from build123d import *

# Parameters (mm, degrees)
CROQUIS2_W              = 31
CROQUIS2_H              = 130
SALIENTE_EXTRUIR1_DEPTH = 69
CROQUIS3_W              = 130
CROQUIS3_H              = 40
SALIENTE_EXTRUIR2_DEPTH = 715
CROQUIS4_W              = 31
CROQUIS4_H              = 130
SALIENTE_EXTRUIR3_DEPTH = 29
CROQUIS7_W              = 684
CROQUIS7_H              = 20
CORTAR_EXTRUIR2_DEPTH   = 125
CROQUIS8_W              = 684
CROQUIS8_H              = 39.960038326
CORTAR_EXTRUIR3_DEPTH   = 1
REDONDEO1_R             = 4


with BuildPart() as part:
    # Croquis2 → Saliente-Extruir1 (new body)
    with BuildSketch(Plane(origin=(0, 0, 0), x_dir=(1, 0, 0), z_dir=(0, 1, 0))):
        with Locations((15.5, 65)):
            Rectangle(CROQUIS2_W, CROQUIS2_H)
    extrude(amount=SALIENTE_EXTRUIR1_DEPTH)

    # Croquis3 → Saliente-Extruir2 (add)
    with BuildSketch(Plane(origin=(31, 0, 0), x_dir=(0, 0, -1), z_dir=(1, 0, 0))):
        with Locations((65, 20)):
            Rectangle(CROQUIS3_W, CROQUIS3_H)
    extrude(amount=SALIENTE_EXTRUIR2_DEPTH)

    # Croquis4 → Saliente-Extruir3 (add)
    with BuildSketch(Plane(origin=(0, 40, 0), x_dir=(1, 0, 0), z_dir=(0, 1, 0))):
        with Locations((730.5, 65)):
            Rectangle(CROQUIS4_W, CROQUIS4_H)
    extrude(amount=SALIENTE_EXTRUIR3_DEPTH)

    # Croquis7 → Cortar-Extruir2 (cut)
    with BuildSketch(Plane(origin=(0, 0, -130), x_dir=(-1, 0, 0), z_dir=(0, 0, -1))):
        with Locations((-373, 30)):
            Rectangle(CROQUIS7_W, CROQUIS7_H)
    extrude(amount=-CORTAR_EXTRUIR2_DEPTH, mode=Mode.SUBTRACT)

    # Croquis8 → Cortar-Extruir3 (cut)
    with BuildSketch(Plane.XY):
        with Locations((373, 20.019980837)):
            Rectangle(CROQUIS8_W, CROQUIS8_H)
    extrude(amount=-CORTAR_EXTRUIR3_DEPTH, mode=Mode.SUBTRACT)

    # Redondeo1
    redondeo1_edges = [part.edges().sort_by_distance(p)[0] for p in [
        (373, 40, -1),
    ]]
    fillet(redondeo1_edges, radius=REDONDEO1_R - 0.0001)  # a hair under: the kernel refuses the full size


solid = part.part
Check sheet for the modelled part. Datum: model origin and axes. Units: mm. A direction names the side the tool comes from. Coordinates: 2 decimals unless noted, no trailing zeros. Write each loop counter-clockwise with the first axis right and the second up, starting at its lowest first coordinate (ties: lowest second). Pieces come first, ordered by that corner, then holes.
Item 1: Cross-section at B-B on z = -45. Record the boundary of the cut face in (x, y).
Numbers:
outline: (0, 0) - (746, 0) - (746, 69) - (715, 69) - (715, 20) - (31, 20) - (31, 69) - (0, 69) - close
Item 2: Access from +Z, -Z, +X, -X, +Y, -Y to the whole of each face (thin tool, end or side, straight path). Record for faces 5 (the face through (378, 20, -68)), 6 (the face through (15, 69, -66)), 7 (the face through (368, 18, -1)).
Numbers:
face 5: -Z, +Y
face 6: +Z, -Z, +X, -X, +Y
face 7: +Z, +Y
Item 3: Scan lines: probe 1 along X at (y, z) = (47, -22); probe 2 along Y at (x, z) = (528.5, -112); probe 3 along Z at (x, y) = (662, 19.5). Record each from-to range of solid material in increasing order.
Numbers:
probe 1: x = 0 to 31, 715 to 746
probe 2: y = 0 to 20
probe 3: z = -130 to -1
Item 4: Cross-section at A-A on y = 49. Record the boundary of the cut face in (x, z), then the cut area to 3 significant figures.
Numbers:
outline: (0, -130) - (31, -130) - (31, 0) - (0, 0) - close; (715, -130) - (746, -130) - (746, 0) - (715, 0) - close
area: 8,060 mm2
Item 5: Mould release check, pull along X, two halves, no side actions. Record for faces 1 (the face through (0, 34, -64)), 2 (the face through (746, 34, -64)), 3 (the face through (12, 34, 0)), 4 (the face through (715, 42, -64)): released by +X, released by -X, zero draft, split by the parting line, or undercut.
Numbers:
face 1: released by -X
face 2: released by +X
face 3: zero draft
face 4: undercut
Item 6: Depth check by flat-ended pin: pin 1 Ø4 at (x, y) = (151.5, 36) entering from -Z; pin 2 Ø3 at (x, y) = (493.5, 18.5) entering from +Z; pin 3 Ø1.5 at (x, z) = (138.5, -101.5) entering from +Y. Enter the tip coordinate at first touch or a pass-through.
Numbers:
pin 1: stops at z = -5
pin 2: stops at z = -1
pin 3: stops at y = 20
